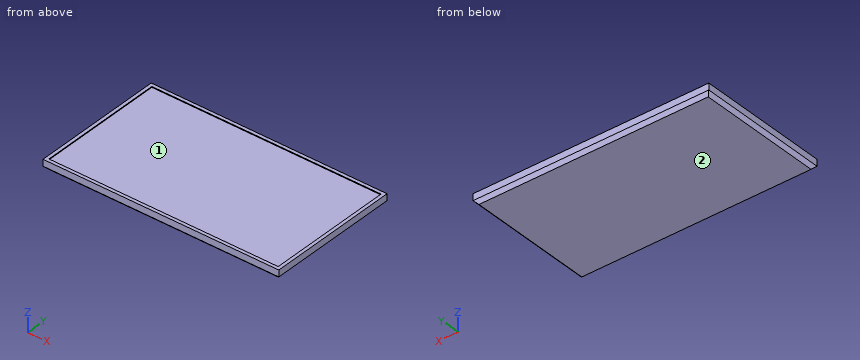
Autodesk Inventor part; units mm, degrees
ref_plane "YZ Plane" through (0, 0, 0) normal (1, 0, 0) x (0, 1, 0)
ref_plane "XZ Plane" through (0, 0, 0) normal (0, 1, 0) x (-1, 0, 0)
ref_plane "XY Plane" through (0, 0, 0) normal (0, 0, 1) x (1, 0, 0)
sketch "Sketch1" plane through (0, 0, 0) normal (0, 0, 1) x (1, 0, 0)
  line L0 (-719.5, -404.5) -> (719.5, -404.5)
  line L1 (719.5, -404.5) -> (719.5, 404.5)
  line L2 (719.5, 404.5) -> (-719.5, 404.5)
  line L3 (-719.5, 404.5) -> (-719.5, -404.5)
  line L4 (-719.5, -404.5) -> (719.5, 404.5) construction
  line L5 (719.5, -404.5) -> (-719.5, 404.5) construction
  point P0 (0, 0)
  dimension "d0" = 1439
  dimension "d1" = 809
extrude "Extrusion1" add sketch "Sketch1" along normal blind 60
shell "Shell1" thickness 20 removed faces 1 at (-239.8333, 134.8333, 60) ; own thickness 55 on faces at (-239.8333, 134.8333, 0)
chamfer "Chamfer1" distance 20 angle 45 4 edges at (719.5, 0, 0) (0, 404.5, 0) (-719.5, 0, 0) (0, -404.5, 0)
properties part number "TV 65"
Verification items for the finished model (mm, model axes). Face numbers are marked on the shaded views. Give positions to 0.01 mm unless a question says otherwise; leave off trailing zeros. Order: outer loops, then holes, each group sorted by start corner. A loop starts at its lowest first (then second) coordinate and runs counter-clockwise, first axis right, second up. Notation, with made-up numbers: M 31.25,17 L 61.25,17 A30 ccw 61.25,54 Z; hole C 41.5,30.25 d4. An arc over 180 degrees is marked long. Answer in a Markdown table with one row per item. Add a question column.
Item 1: Section check A-A, the plane x = 327.5. Enter the section's corners in (y, z).
Item 2: Scan lines: probe 1 along X at (y, z) = (322.5, 55.5); probe 2 along Z at (x, y) = (339, 59); probe 3 along X at (y, z) = (354, 19.5). Record each from-to range of solid material in increasing order. Write a range as from..to.
Item 3: Section check B-B, the plane y = -113. Enter the section's corners in (x, z), and give its area (3 significant figures).
Item 4: Mould release check, pull along Y, two halves, no side actions. Record for the marked faces 1 and 2: released by +Y, released by -Y, zero draft, split by the parting line, or undercut.
Filled sheet:
| question | item | result |
|---|---|---|
| 1 | outline | M -404.5,20 L -384.5,0 L 384.5,0 L 404.5,20 L 404.5,60 L 384.5,60 L 384.5,55 L -384.5,55 L -384.5,60 L -404.5,60 Z |
| 2 | probe 1 | x = -719.5..-699.5, 699.5..719.5 |
| 2 | probe 2 | z = 0..55 |
| 2 | probe 3 | x = -719..719 |
| 3 | outline | M -719.5,20 L -699.5,0 L 699.5,0 L 719.5,20 L 719.5,60 L 699.5,60 L 699.5,55 L -699.5,55 L -699.5,60 L -719.5,60 Z |
| 3 | area | 78,900 mm^2 |
| 4 | face 1 | undercut |
| 4 | face 2 | zero draft |
